Build history of the part. All positions in model axes, mm. A direction names the side the tool comes from. Give positions to 0.01 mm unless a question says otherwise; leave off trailing zeros. Order: outer loops, then holes, each group sorted by start corner. A loop starts at its lowest first (then second) coordinate and runs counter-clockwise, first axis right, second up. Notation, with made-up numbers: (-37, -36.75) - (5, -36.75) arc R19 cw to (5, -5.75) - close; hole circle Ø6 at (88, -30.75). An arc over 180 degrees is marked (long way). Answer in a Markdown table with one row per item.
```python
from build123d import *

# Parameters (mm, degrees)
BOSS_EXTRUDE1_DEPTH = 1.5
BOSS_EXTRUDE2_DEPTH = 81
BOSS_EXTRUDE3_DEPTH = 3


with BuildPart() as part:
    # Sketch1 → Boss-Extrude1 (new, symmetric)
    with BuildSketch(Plane.XY):
        with BuildLine():
            Line((31.56, -47.50625778), (31.56, 71.89374222))
            Line((31.56, 71.89374222), (-11.5, 71.89374222))
            ThreePointArc((-11.5, 71.89374222), (-25.642135624, 66.035877844), (-31.5, 51.89374222))
            Line((-31.5, 51.89374222), (-31.5, -67.60625778))
            ThreePointArc((-31.5, -67.60625778), (-30.035533906, -71.141791686), (-26.5, -72.60625778))
            Line((-26.5, -72.60625778), (-20.24, -72.60625778))
            ThreePointArc((-20.24, -72.60625778), (-16.704466094, -71.141791686), (-15.24, -67.60625778))
            Line((-15.24, -67.60625778), (-15.24, -38.60625778))
            ThreePointArc((-15.24, -38.60625778), (-13.775533906, -35.070723874), (-10.24, -33.60625778))
            Line((-10.24, -33.60625778), (8.26, -33.60625778))
            ThreePointArc((8.26, -33.60625778), (11.795533906, -35.070723874), (13.26, -38.60625778))
            Line((13.26, -38.60625778), (13.26, -42.50625778))
            ThreePointArc((13.26, -42.50625778), (14.724466094, -46.041791686), (18.26, -47.50625778))
            Line((18.26, -47.50625778), (31.56, -47.50625778))
        make_face()
    extrude(amount=BOSS_EXTRUDE1_DEPTH, both=True)

    # Sketch2 → Boss-Extrude2 (add)
    with BuildSketch(Plane(origin=(0, 0, -1.5), x_dir=(-1, 0, 0), z_dir=(0, 0, -1))):
        with BuildLine():
            Line((28.5, -67.60625778), (28.5, 51.89374222))
            ThreePointArc((28.5, 51.89374222), (23.52081528, 63.9145575), (11.5, 68.89374222))
            Line((11.5, 68.89374222), (-28.56, 68.89374222))
            Line((-28.56, 68.89374222), (-31.56, 68.89374222))
            Line((-31.56, 68.89374222), (-31.56, 71.89374222))
            Line((-31.56, 71.89374222), (11.5, 71.89374222))
            ThreePointArc((11.5, 71.89374222), (25.642135624, 66.035877844), (31.5, 51.89374222))
            Line((31.5, 51.89374222), (31.5, -67.60625778))
            ThreePointArc((31.5, -67.60625778), (30.683300133, -70.344870568), (28.5, -72.188833475))
            Line((28.5, -72.188833475), (28.5, -67.60625778))
        make_face()
    extrude(amount=BOSS_EXTRUDE2_DEPTH)

    # Sketch3 → Boss-Extrude3 (add)
    with BuildSketch(Plane(origin=(0, 0, -82.5), x_dir=(-1, 0, 0), z_dir=(0, 0, -1))):
        with BuildLine():
            Line((-31.56, 68.89374222), (-31.56, 71.89374222))
            Line((-31.56, 71.89374222), (11.5, 71.89374222))
            ThreePointArc((11.5, 71.89374222), (25.642135624, 66.035877844), (31.5, 51.89374222))
            Line((31.5, 51.89374222), (31.5, -67.60625778))
            ThreePointArc((31.5, -67.60625778), (30.683300133, -70.344870568), (28.5, -72.188833475))
            ThreePointArc((28.5, -72.188833475), (27.521548218, -72.500789345), (26.5, -72.60625778))
            Line((26.5, -72.60625778), (20.24, -72.60625778))
            ThreePointArc((20.24, -72.60625778), (16.704466094, -71.141791686), (15.24, -67.60625778))
            Line((15.24, -67.60625778), (15.24, -38.60625778))
            ThreePointArc((15.24, -38.60625778), (13.775533906, -35.070723874), (10.24, -33.60625778))
            Line((10.24, -33.60625778), (-8.26, -33.60625778))
            ThreePointArc((-8.26, -33.60625778), (-11.795533906, -35.070723874), (-13.26, -38.60625778))
            Line((-13.26, -38.60625778), (-13.26, -42.50625778))
            ThreePointArc((-13.26, -42.50625778), (-14.724466094, -46.041791686), (-18.26, -47.50625778))
            Line((-18.26, -47.50625778), (-31.56, -47.50625778))
            Line((-31.56, -47.50625778), (-31.56, 68.89374222))
        make_face()
    extrude(amount=BOSS_EXTRUDE3_DEPTH)


solid = part.part
```
1. Cut at A-A on y = 44.5. Write the cut outline in (x, z).
Check result:
| item | result |
|---|---|
| outline | (-31.5, -85.5) - (31.56, -85.5) - (31.56, -82.5) - (-28.5, -82.5) - (-28.5, -1.5) - (31.56, -1.5) - (31.56, 1.5) - (-31.5, 1.5) - close |
2. Probe line 1 (Z direction, x = 0, y = 3.5); line 2 (Y direction, x = -1, z = -4.5); line 3 (X direction, y = 44.5, z = -9.5). List the from-to ranges inside material, lowest first.
Check result:
| item | result |
|---|---|
| line 1 | z = -85.5 to -82.5, -1.5 to 1.5 |
| line 2 | y = 68.89 to 71.89 |
| line 3 | x = -31.5 to -28.5 |
3. Two-plate mould, pull along X, no slides. Class faces 1 (the face through (11.756, -35.032, -83.979)), 2 (the face through (10, 68.894, -41)), 3 (the face through (-28.5, -11, -41)): +X half, -X half, draft (parallel to the pull), parting line (faces both ways), or undercut.
Check result:
| item | result |
|---|---|
| face 1 | undercut |
| face 2 | draft |
| face 3 | +X half |
4. Which spindle directions (+Z, -Z, +X, -X, +Y, -Y) get a long thin tool onto all of the face, cutting with end or side? Do faces 4 (the face through (10, 71.894, -41)), 5 (the face through (-1, -33.606, 0)), 6 (the face through (-23.652, 63.782, -41.433)), 7 (the face through (25, -47.506, -84)). Say none if no direction does.
Check result:
| item | result |
|---|---|
| face 4 | +Z, -Z, +X, -X, +Y |
| face 5 | +Z, -Z, -Y |
| face 6 | +X, -Y |
| face 7 | +Z, -Z, +X, -Y |
5. Drop flat-ended pins along their axis: P1, Ø2.5, axis at x = 23.5, z = -0.5, coming from the -Y side; P2, Ø2.5, axis at y = -52.5, z = 0.5, coming from the +X side; P3, Ø4, axis at y = -32, z = -56, coming from the +X side. Give the stop position or say it passes through.
Check result:
| item | result |
|---|---|
| P1 | stops at y = -47.51 |
| P2 | stops at x = -15.24 |
| P3 | stops at x = -28.5 |
6. Cut at B-B on x = -0.5. Write the cut outline in (y, z).
Check result:
| item | result |
|---|---|
| outline | (-33.61, -85.5) - (71.89, -85.5) - (71.89, 1.5) - (-33.61, 1.5) - (-33.61, -1.5) - (68.89, -1.5) - (68.89, -82.5) - (-33.61, -82.5) - close |
